```python
from build123d import *

# Parameters (mm, degrees)
SKETCH_1_W          = 60
SKETCH_1_H          = 14
EXTRUDE_1_DEPTH     = 20
SKETCH_2_W          = 20
SKETCH_2_H          = 8
CUT_EXTRUDE_1_DEPTH = 15
SKETCH_3_R          = 1.5
CUT_EXTRUDE_2_DEPTH = 10.5
FILLET_1_R          = 5
SKETCH_4_R          = 2
CUT_EXTRUDE_3_DEPTH = 21
CHAMFER_1_SIZE      = 2
SKETCH_5_R          = 5.4
SKETCH_5_R_2        = 2
EXTRUDE_2_DEPTH     = 5.5


with BuildPart() as part:
    # Эскиз1 → Бобышка-Вытянуть1 (new body)
    with BuildSketch(Plane.XY):
        Rectangle(SKETCH_1_W, SKETCH_1_H)
    extrude(amount=EXTRUDE_1_DEPTH)

    # Эскиз2 → Вырез-Вытянуть1 (cut, through all)
    with BuildSketch(Plane(origin=(0, -7, 0), x_dir=(-1, 0, 0), z_dir=(0, -1, 0))):
        with Locations((0, -12.5)):
            Rectangle(SKETCH_2_W, SKETCH_2_H)
    extrude(amount=-CUT_EXTRUDE_1_DEPTH, mode=Mode.SUBTRACT)

    # Эскиз3 → Вырез-Вытянуть2 (cut)
    with BuildSketch(Plane(origin=(0, 7, 0), x_dir=(1, 0, 0), z_dir=(0, 1, 0))):
        with Locations((-21, -12.5)):
            Circle(SKETCH_3_R)
        with Locations((21, -12.5)):
            Circle(SKETCH_3_R)
    extrude(amount=-CUT_EXTRUDE_2_DEPTH, mode=Mode.SUBTRACT)

    # Скругление1
    fillet_1_edges = [part.edges().sort_by_distance(p)[0] for p in [
        (30, 0, 20),
        (-30, 0, 20),
    ]]
    fillet(fillet_1_edges, radius=FILLET_1_R)

    # Эскиз4 → Вырез-Вытянуть3 (cut, through all)
    with BuildSketch(Plane.XY.offset(20)):
        with Locations((24.6, 0)):
            Circle(SKETCH_4_R)
        with Locations((-24.6, 0)):
            Circle(SKETCH_4_R)
        Circle(SKETCH_4_R)
    extrude(amount=-CUT_EXTRUDE_3_DEPTH, mode=Mode.SUBTRACT)

    # Фаска1
    chamfer_1_edges = [part.edges().sort_by_distance(p)[0] for p in [
        (-2, 0, 20),
    ]]
    chamfer(chamfer_1_edges, length=CHAMFER_1_SIZE)

    # Эскиз5 → Бобышка-Вытянуть2 (add)
    with BuildSketch(Plane.XY.offset(20)):
        with Locations((-24.6, 0)):
            Circle(SKETCH_5_R)
        with Locations((-24.6, 0)):
            Circle(SKETCH_5_R_2, mode=Mode.SUBTRACT)
        with Locations((24.6, 0)):
            Circle(SKETCH_5_R)
        with Locations((24.6, 0)):
            Circle(SKETCH_5_R_2, mode=Mode.SUBTRACT)
    extrude(amount=-EXTRUDE_2_DEPTH)


solid = part.part
```
CAD build for the part. Positions are in the model's coordinates, mm. A direction names the side the tool comes from. Round coordinates to 2 decimals unless told otherwise and drop trailing zeros. Order: outer loops, then holes, each group sorted by start corner. A loop starts at its lowest first (then second) coordinate and runs counter-clockwise, first axis right, second up. Notation, with made-up numbers: (60.25, -35) - (98.25, -35) arc R27 cw to (98.25, -4) - close; hole circle Ø2 at (49.5, 7). An arc over 180 degrees is marked (long way). Use CSV: the item, a comma, the result in double quotes. Start each with the question number.
1) Two-plate mould, pull along X, no slides. Class faces 6 (the flat face through (-10, 0, 13)), 7 (the cylindrical face through (-29, -5, 18)), 8 (the cylindrical face through (29, -5, 18)): pulls with the +X half, pulls with the -X half, needs draft (parallel to the pull), parting line crosses it, or undercut.
2) Tool access for faces 1 (the flat face through (2.4, -0.1, 16.5)), 2 (the cylindrical face through (29, 5, 18)), 3 (the cylindrical face through (-30, 0, 19)), 4 (the cylindrical face through (-29, 5, 18)), 5 (the cylindrical face through (19.5, 1.82, 12.43)): list every direction of +Z, -Z, +X, -X, +Y, -Y with a clear straight run to the whole face (end or side of a thin tool).
3) Saw through at B-B (x = 7). List the corners of the cut face in (y, z), and give its area (3 significant figures).
4) Saw through at C-C (y = 6). List the corners of the cut face in (x, z), and give its area (3 significant figures).
5) Pin check, flat tips, straight feed: pin 1 Ø2.5 at (x, y) = (24.6, 0) entering from -Z; pin 2 Ø4 at (x, y) = (-1.5, -0.5) entering from +Z; pin 3 Ø1.8 at (x, z) = (21, 12.5) entering from +Y. Stop position of each tip, or through.
6) Wall check: L1, parallel to X at y = 4, z = 12.5; L2, parallel to Z at x = 8.5, y = 6; L3, parallel to Y at x = -24.6, z = 11.5. Give the ranges that are in metal, low to high. Write a range as [from, to].
7) Saw through at D-D (z = 10). List the corners of the cut face in (x, y).
8) Saw through at A-A (z = 12.5). List the corners of the cut face in (x, y), and give its area (3 significant figures).
Values follow:
1,face 6,"undercut"
1,face 7,"pulls with the -X half"
1,face 8,"pulls with the +X half"
2,face 1,"+Y, -Y"
2,face 2,"+Z, +X, +Y"
2,face 3,"+Z, -X"
2,face 4,"+Z, -X, +Y"
2,face 5,"+Y"
3,outline,"(-7, 0) - (7, 0) - (7, 8.5) - (-7, 8.5) - close; (-7, 16.5) - (7, 16.5) - (7, 20) - (-7, 20) - close"
3,area,"168 mm2"
4,outline,"(-30, 0) - (30, 0) - (30, 15) arc R5 ccw to (25, 20) - (-25, 20) arc R5 ccw to (-30, 15) - close; hole circle Ø3 at (-21, 12.5); hole (-10, 8.5) - (10, 8.5) - (10, 16.5) - (-10, 16.5) - close; hole circle Ø3 at (21, 12.5)"
4,area,"1,020 mm2"
5,pin 1,"passes through"
5,pin 2,"stops at z = 19.58"
5,pin 3,"stops at y = -3.5"
6,L1,"x = [-30, -22.5], [-19.5, -10], [10, 19.5], [22.5, 30]"
6,L2,"z = [0, 8.5], [16.5, 20]"
6,L3,"y = [-7, -2], [2, 7]"
7,outline,"(-30, -7) - (-10, -7) - (-10, 7) - (-30, 7) - close; (10, -7) - (30, -7) - (30, 7) - (10, 7) - close; hole circle Ø4 at (-24.6, 0); hole circle Ø4 at (24.6, 0)"
8,outline,"(-30, -7) - (-10, -7) - (-10, 7) - (-19.5, 7) - (-19.5, -3.5) - (-22.5, -3.5) - (-22.5, 7) - (-30, 7) - close; (10, -7) - (30, -7) - (30, 7) - (22.5, 7) - (22.5, -3.5) - (19.5, -3.5) - (19.5, 7) - (10, 7) - close; hole circle Ø4 at (-24.6, 0); hole circle Ø4 at (24.6, 0)"
8,area,"472 mm2"
